from build123d import *

# Parameters (mm, degrees)
SKETCH1_R           = 24.13
SKETCH1_R_2         = 2.5
SKETCH1_R_3         = 6.35
BOSS_EXTRUDE1_DEPTH = 3.175


with BuildPart() as part:
    # Sketch1 → Boss-Extrude1 (new body)
    with BuildSketch(Plane(origin=(0, 0, 0), x_dir=(1, 0, 0), z_dir=(0, 1, 0))):
        Circle(SKETCH1_R)
        with Locations((19.2, 0)):
            Circle(SKETCH1_R_2, mode=Mode.SUBTRACT)
        with Locations((-9.6, 16.627687753)):
            Circle(SKETCH1_R_2, mode=Mode.SUBTRACT)
        with Locations((-9.6, -16.627687753)):
            Circle(SKETCH1_R_2, mode=Mode.SUBTRACT)
        Circle(SKETCH1_R_3, mode=Mode.SUBTRACT)
    extrude(amount=BOSS_EXTRUDE1_DEPTH)


solid = part.part
For this review, take the finished solid that the model builds, in its own axes (mm). Round coordinates to 2 decimals unless told otherwise and drop trailing zeros. Write each loop counter-clockwise with the first axis right and the second up, starting at its lowest first coordinate (ties: lowest second). Pieces come first, ordered by that corner, then holes. Notation, with made-up numbers: (-20.75, 23.25) - (5.25, 23.25) arc R24 ccw to (5.25, 59.25) - close; hole circle Ø9 at (5.25, -36.75). An arc over 180 degrees is marked (long way). Use a Markdown table: item, result.
Q1. The part is to be moulded in two halves that separate along Z. For faces 1 (the cylindrical face through (23.016, 1.565, -7.248)), 2 (the cylindrical face through (-8.446, 1.565, 18.846)), 3 (the flat face through (5, 3.175, 5)), say which applies: pulls with the +Z half, pulls with the -Z half, needs draft (parallel to the pull), parting line crosses it, or undercut.
Derived:
| item | result |
|---|---|
| face 1 | parting line crosses it |
| face 2 | undercut |
| face 3 | needs draft |
Q2. We need section B-B (z = 0). Give the boundary of the cut face in (x, y) (3 decimals).
Derived:
| item | result |
|---|---|
| outline | (-24.13, 0) - (-6.35, 0) - (-6.35, 3.175) - (-24.13, 3.175) - close; (6.35, 0) - (16.7, 0) - (16.7, 3.175) - (6.35, 3.175) - close; (21.7, 0) - (24.13, 0) - (24.13, 3.175) - (21.7, 3.175) - close |
Q3. We need section A-A (x = 0). Give the boundary of the cut face in (y, z) (3 decimals).
Derived:
| item | result |
|---|---|
| outline | (0, -24.13) - (3.175, -24.13) - (3.175, -6.35) - (0, -6.35) - close; (0, 6.35) - (3.175, 6.35) - (3.175, 24.13) - (0, 24.13) - close |
Q4. Clearance check with flat-ended pins moving along their axes: pin 1 (1.5 mm diameter, centred on y = 2, z = -2, fed in from -X); pin 2 (3 mm diameter, centred on x = 19.2, z = 0, fed in from -Y); pin 3 (2 mm diameter, centred on x = -17, z = -10, fed in from -Y). State where each tip first meets the part, or that it passes through.
Derived:
| item | result |
|---|---|
| pin 1 | stops at x = -24.1 |
| pin 2 | passes through |
| pin 3 | stops at y = 0 |
Q5. We need section D-D (x = 19.2). Give the boundary of the cut face in (y, z) (3 decimals), plus the area to 3 significant figures.
Derived:
| item | result |
|---|---|
| outline | (0, -14.616) - (3.175, -14.616) - (3.175, -2.5) - (0, -2.5) - close; (0, 2.5) - (3.175, 2.5) - (3.175, 14.616) - (0, 14.616) - close |
| area | 76.9 mm2 |
Q6. We need section C-C (y = 1.65). Give the boundary of the cut face in (x, z), plus the area to 3 significant figures.
Derived:
| item | result |
|---|---|
| outline | circle Ø48.26 at (0, 0); hole circle Ø5 at (-9.6, -16.63); hole circle Ø5 at (-9.6, 16.63); hole circle Ø12.7 at (0, 0); hole circle Ø5 at (19.2, 0) |
| area | 1,640 mm2 |
Q7. Wall thickness on line 1 along X through (y, z) = (2.2, 2); line 2 along Z through (x, y) = (0, 0.85); line 3 along Z through (x, y) = (-9.6, 2.05): over which ranges is each line inside the solid? List them lowest first.
Derived:
| item | result |
|---|---|
| line 1 | x = -24.05 to -6.03, 6.03 to 17.7, 20.7 to 24.05 |
| line 2 | z = -24.13 to -6.35, 6.35 to 24.13 |
| line 3 | z = -22.14 to -19.13, -14.13 to 14.13, 19.13 to 22.14 |
